Work out the finished part from the listing and answer in its coordinate system (mm). Face numbers are marked on the shaded views. A direction names the side the tool comes from. Coordinates: 2 decimals unless noted, no trailing zeros. Order: outer loops, then holes, each group sorted by start corner. A loop starts at its lowest first (then second) coordinate and runs counter-clockwise, first axis right, second up. Notation, with made-up numbers: (11, 77.25) -> (19, 77.25) arc R16 ccw to (19, 85.25) -> close; hole circle Ø2 at (30.5, -30). An arc over 180 degrees is marked (long way). Write item = value, one per line. Start each with the question number.
Q1. For a pull along Y with two mould halves and no side action, classify the marked faces 4, 5 and 6 as +Y half, -Y half, draft (parallel to the pull), parting line (faces both ways), or undercut.
Q2. Which of the six approach directions +Z, -Z, +X, -X, +Y, -Y give full straight-line access (tool end or side, diameter ignored) to the marked faces 1, 2 and 3?
Q3. Straight lines are drawn through the part: L1, parallel to Y at x = -2.2, z = -2.2; L2, parallel to X at y = 35, z = -1.85; L3, parallel to Y at x = -4.25, z = -3.1. For each, find the intervals that lie inside material, in ascending order. Write a range as from..to.
Q4. The part is cut by section A-A, the plane x = -13. Determine the outline of the cut face in (y, z).
Q5. The part is cut by section D-D, the plane y = 39.75. Determine the outline of the cut face in (x, z).
Q6. Flat-ended cylindrical pins translate along their axes: pin 1 (4 mm diameter, centred on x = -10, y = 30.5, fed in from +Z); pin 2 (1.9 mm diameter, centred on x = -9.5, z = -1, fed in from -Y); pin 3 (2 mm diameter, centred on x = -11.5, y = 34.5, fed in from +Z); pin 4 (2 mm diameter, centred on y = 32.5, z = -2, fed in from +X). Find the tip coordinate at first contact, or state that the pin passes through.
Q7. The part is cut by section C-C, the plane x = -5.5. Determine the outline of the cut face in (y, z), plus the area to 3 significant figures.
Q8. The part is cut by section B-B, the plane z = -0.85. Determine the outline of the cut face in (x, y), plus the area to 3 significant figures.
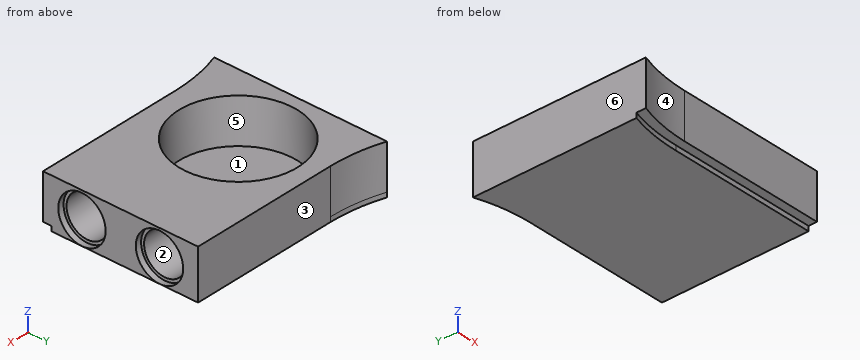
Autodesk Inventor part; units mm, degrees
ref_plane "YZ Plane" through (0, 0, 0) normal (1, 0, 0) x (0, 1, 0)
ref_plane "XZ Plane" through (0, 0, 0) normal (0, 1, 0) x (-1, 0, 0)
ref_plane "XY Plane" through (0, 0, 0) normal (0, 0, 1) x (1, 0, 0)
sketch "Sketch1" plane through (0, 0, 0) normal (0, 0, 1) x (1, 0, 0)
  circle A0 centre (-14.5, 55.2958) radius 13.85
  circle A1 centre (-14.5, 55.2958) radius 14.5
  circle A2 centre (-14.5, 14.5) radius 13.85
  circle A3 centre (-14.5, 14.5) radius 14.5
  circle A4 centre (-13, 35.0012) radius 5
  line L0 (0, 65.2958) -> (-19, 65.2958)
  line L1 (-19, 65.2958) -> (-19, -1.7042)
  line L2 (-19, -1.7042) -> (0, -1.7042)
  line L3 (0, -1.7042) -> (0, 65.2958)
  line L4 (-2, 65.2958) -> (-2, -1.7042)
  line L5 (-14.5, 41.4458) -> (-2, 41.4458)
  line L6 (-14.5, 40.7958) -> (-2, 40.7958)
  line L7 (-14.5, 28.35) -> (-2, 28.35)
  line L8 (-14.5, 29) -> (-2, 29)
  point P0 (0, 0)
  point P1 (-19, 42.1973)
  point P2 (-19, 27.5986)
  point P3 (-19, 28.284)
  point P4 (-19, 41.5118)
  dimension "d0" = 67
  dimension "d1" = 1
  dimension "d2" = 2
extrude "Extrusion1" add sketch "Sketch1" against normal blind 3.8 contours L5 A1 L1 A0 | L5 L4 L6 A1 | A1 L6 L4 L8 A3 L1 | A3 L7 A2 L1 | L4 L7 A3 L8
ref_plane "Work Plane7" through (0, 0, -3.8) normal (0, 0, -1) x (-1, 0, 0)
sketch "Sketch2" plane through (0, 0, -3.8) normal (0, 0, -1) x (-1, 0, 0)
  circle A0 centre (8.5216, 9.2187) radius 1.0564
  circle A1 centre (20.7784, 19.5033) radius 1.0564
  circle A2 centre (14.65, 14.361) radius 5
  circle A3 centre (14.65, 14.361) radius 14
  circle A4 centre (14.65, 14.361) radius 14.7
  line L0 (2, 41.4458) -> (2, 28.35)
  line L1 (2, 28.35) -> (14.5, 28.35)
  arc A5 (19, 27.5986) -> (14.5, 28.35) centre (14.5, 14.5) ccw
  line L2 (19, 27.5986) -> (19, 42.1973)
  arc A6 (14.5, 41.4458) -> (19, 42.1973) centre (14.5, 55.2958) ccw
  line L3 (14.5, 41.4458) -> (2, 41.4458)
  circle A7 centre (13, 35.0012) radius 5
  line L4 (14.5, 29.0603) -> (2, 29.0603)
  line L5 (2, 41.4458) -> (2, 28.35)
  line L6 (14.5, 29.0603) -> (14.5, 14.5)
  point P0 (0, 0)
  point P1 (2, 29.0603)
  point P2 (19, 28.4027)
extrude "Extrusion4" add sketch "Sketch2" along normal blind 0.4 contours A4 L4 L0 L3 A6 L2 | A7
sketch "Sketch3" plane through (-2, 28.35, 0) normal (1, 0, 0) x (0, 0, -1)
  line L0 (0, 0) -> (0, 13.0958)
  line L1 (0, 0) -> (3.8, 0)
  line L2 (0, 6.5784) -> (4.4, 6.5784)
  line L3 (0, 13.0958) -> (4.4, 6.5784)
  line L4 (4.4, 6.5784) -> (0, 0)
  line L5 (0, 6.5784) -> (2.2, 3.2892)
  line L6 (0, 6.5784) -> (2.2, 9.8371)
  line L7 (0, 13.0958) -> (4.2, 13.0958)
  line L8 (3.8, 0.7103) -> (3.8, 0)
  line L9 (3.8, 0.7103) -> (4.2, 0.7103)
  line L10 (4.2, 13.0958) -> (4.2, 0.7103)
  point P0 (0, -28.35)
  point P1 (5.9, 0.65)
  point P2 (5.9, 12.4458)
  dimension "d12" = 6.5784
hole "Hole1" at (-2, 38.1871, -2.2) at (-2, 31.6392, -2.2) direction (-1, 0, 0) diameter 3.5 depth 4.5 counterbore diameter 4 counterbore depth 0.5
properties part number "BearigHoldRight"
Model answer:
q1.face_4 = -Y half
q1.face_5 = undercut
q1.face_6 = draft
q2.face_1 = +Z
q2.face_2 = +X
q2.face_3 = +Z, -Z, +X, +Y
q3.L1 = 28.35..29.64, 33.64..36.19, 40.19..41.45
q3.L2 = -19..-18, -8..-2
q3.L3 = 28.35..30.14, 33.14..36.69, 39.69..41.45
q4.outline = (28.35, -3.8) -> (29.06, -3.8) -> (29.06, -4.2) -> (41.45, -4.2) -> (41.45, 0) -> (40, 0) -> (40, -3.8) -> (30, -3.8) -> (30, 0) -> (28.35, 0) -> close
q5.outline = (-19, -4.2) -> (-2, -4.2) -> (-2, -3.45) -> (-2.5, -3.45) -> (-2.5, -2.99) -> (-6.5, -2.99) -> (-6.5, -1.41) -> (-2.5, -1.41) -> (-2.5, -0.95) -> (-2, -0.95) -> (-2, 0) -> (-11.44, 0) -> (-11.44, -3.8) -> (-14.56, -3.8) -> (-14.56, 0) -> (-19, 0) -> close
q6.pin_1 = 0
q6.pin_2 = 28.35
q6.pin_3 = -3.8
q6.pin_4 = -2.5
q7.outline = (28.35, -3.8) -> (29.06, -3.8) -> (29.06, -4.2) -> (41.45, -4.2) -> (41.45, 0) -> (28.35, 0) -> close; hole circle Ø3.5 at (31.64, -2.2); hole circle Ø3.5 at (38.19, -2.2)
q7.area = 35.5 mm2
q8.outline = (-19, 27.6) arc R13.85 cw to (-14.5, 28.35) -> (-2, 28.35) -> (-2, 30.16) -> (-2.5, 30.16) -> (-2.5, 30.53) -> (-6.5, 30.53) -> (-6.5, 32.75) -> (-2.5, 32.75) -> (-2.5, 33.11) -> (-2, 33.11) -> (-2, 36.71) -> (-2.5, 36.71) -> (-2.5, 37.07) -> (-6.5, 37.07) -> (-6.5, 39.3) -> (-2.5, 39.3) -> (-2.5, 39.66) -> (-2, 39.66) -> (-2, 41.45) -> (-14.5, 41.45) arc R13.85 cw to (-19, 42.2) -> close; hole circle Ø10 at (-13, 35)
q8.area = 126 mm2
